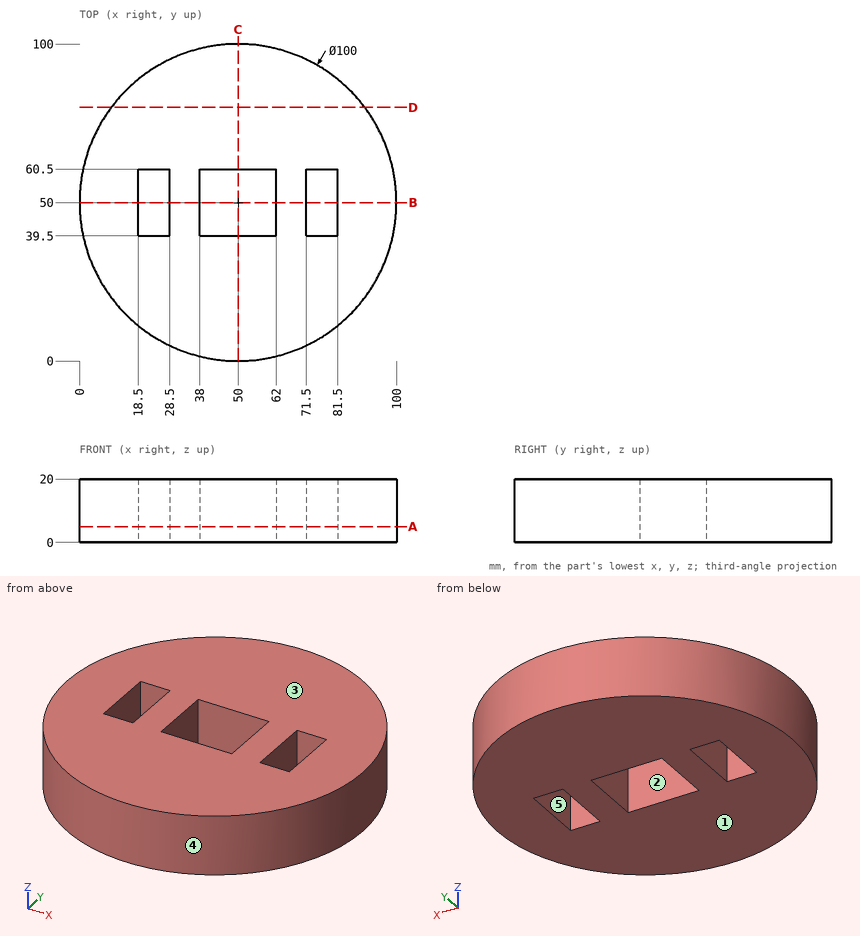
Verification items for this drawing (mm, ordinates from the low corner). A direction names the side the tool comes from. Coordinates: 2 decimals unless noted, no trailing zeros. Order: outer loops, then holes, each group sorted by start corner. A loop starts at its lowest first (then second) coordinate and runs counter-clockwise, first axis right, second up. Notation, with made-up numbers: (66.25, -10.75) -> (80.25, -10.75) arc R8 ccw to (80.25, -6.75) -> close; hole circle Ø11 at (-38, 59.5). An arc over 180 degrees is marked (long way). Put each result on its own line as item: value. Start each with the question number.
1. Access from +Z, -Z, +X, -X, +Y, -Y to the whole of each face (thin tool, end or side, straight path). Record for the marked faces 1 and 2.
2. Cross-section at C-C, the plane x = 50. Record the boundary of the cut face in (y, z), then the cut area to 3 significant figures.
3. Cross-section at A-A, the plane z = 5. Record the boundary of the cut face in (x, y), then the cut area to 3 significant figures.
4. Mould release check, pull along Y, two halves, no side actions. Record for the marked faces 3, 4 and 5: released by +Y, released by -Y, zero draft, split by the parting line, or undercut.
5. Cross-section at B-B, the plane y = 50. Record the boundary of the cut face in (x, z), then the cut area to 3 significant figures.
6. Material ranges on L1, parallel to X at y = 48, z = 4; L2, parallel to X at y = 59.5, z = 15.25; L3, parallel to Y at x = 72, z = 9, recorded low to high. Write a range as [from, to].
7. Go/stop test with flat-tipped pins: pin 1 Ø11 at (x, z) = (22.5, 13.5) entering from +Y; pin 2 Ø8 at (y, z) = (18.5, 5) entering from -X; pin 3 Ø6 at (x, z) = (53.5, 11.5) entering from -Y. Record where each tip stops, or that it passes through.
8. Cross-section at D-D, the plane y = 80. Record the boundary of the cut face in (x, z).
Computed:
1. face 1: -Z, +X, -X, +Y, -Y
1. face 2: +Z, -Z
2. outline: (0, 0) -> (39.5, 0) -> (39.5, 20) -> (0, 20) -> close; (60.5, 0) -> (100, 0) -> (100, 20) -> (60.5, 20) -> close
2. area: 1,580 mm2
3. outline: circle Ø100 at (50, 50); hole (18.5, 39.5) -> (28.5, 39.5) -> (28.5, 60.5) -> (18.5, 60.5) -> close; hole (38, 39.5) -> (62, 39.5) -> (62, 60.5) -> (38, 60.5) -> close; hole (71.5, 39.5) -> (81.5, 39.5) -> (81.5, 60.5) -> (71.5, 60.5) -> close
3. area: 6,930 mm2
4. face 3: zero draft
4. face 4: split by the parting line
4. face 5: undercut
5. outline: (0, 0) -> (18.5, 0) -> (18.5, 20) -> (0, 20) -> close; (28.5, 0) -> (38, 0) -> (38, 20) -> (28.5, 20) -> close; (62, 0) -> (71.5, 0) -> (71.5, 20) -> (62, 20) -> close; (81.5, 0) -> (100, 0) -> (100, 20) -> (81.5, 20) -> close
5. area: 1,120 mm2
6. L1: [0.04, 18.5], [28.5, 38], [62, 71.5], [81.5, 99.96]
6. L2: [0.91, 18.5], [28.5, 38], [62, 71.5], [81.5, 99.09]
6. L3: [5.1, 39.5], [60.5, 94.9]
7. pin 1: y = 94.9
7. pin 2: x = 8.24
7. pin 3: y = 0
8. outline: (10, 0) -> (90, 0) -> (90, 20) -> (10, 20) -> close
